Work out the finished part from the listing and answer in its coordinate system (mm). Face numbers are marked on the shaded views. Give positions to 0.01 mm unless a question says otherwise; leave off trailing zeros. Loops run counter-clockwise (first coordinate to the right, second up) from the corner with the lowest first, then second, coordinate; pieces in that order, holes last. Notation, with made-up numbers: (79, 27) - (108, 27) arc R11 ccw to (108, 35) - close; hole circle Ø7 at (-16, -10.5). An arc over 180 degrees is marked (long way). One line per item, written item: value.
from build123d import *

# Parameters (mm, degrees)
F0_W     = 40.64
F0_H     = 21.59
F1_DEPTH = 1.905
F2_R     = 5.08


with BuildPart() as f1:
    # F0 (on Front) → F1 (new body, symmetric)
    with BuildSketch(Plane.XZ):
        with Locations((-13.928885, -27.195361)):
            Rectangle(F0_W, F0_H)
    extrude(amount=F1_DEPTH, both=True)

    # F2
    f2_edges = [f1.edges().sort_by_distance(p)[0] for p in [
        (-34.248885, 0, -16.400361),
        (6.391115, 0, -16.400361),
        (-34.248885, 0, -37.990361),
        (6.391115, 0, -37.990361),
    ]]
    fillet(f2_edges, radius=F2_R)


solid = f1.part
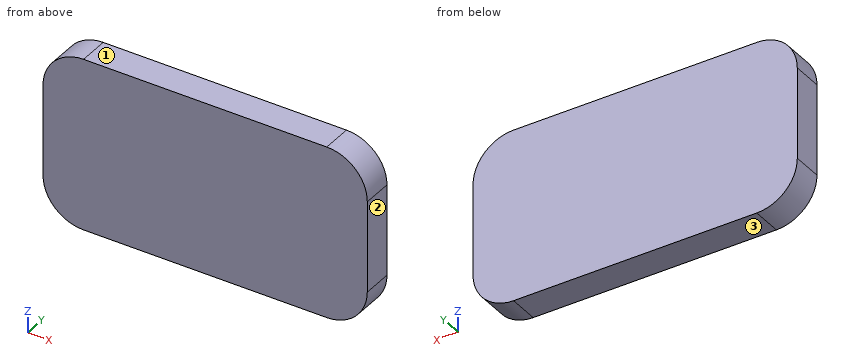
1. Section A-A (y = -0.5) is taken. Write down the section's boundary in (x, z).
Output:
outline: (-34.25, -32.91) arc R5.08 ccw to (-29.17, -37.99) - (1.31, -37.99) arc R5.08 ccw to (6.39, -32.91) - (6.39, -21.48) arc R5.08 ccw to (1.31, -16.4) - (-29.17, -16.4) arc R5.08 ccw to (-34.25, -21.48) - close
2. The mould has two halves that part along Z. Classify the marked faces 1, 2 and 3: released by +Z, released by -Z, zero draft, split by the parting line, or undercut.
Output:
face 1: released by +Z
face 2: zero draft
face 3: released by -Z
3. Find the intervals of material crossed by line 1 along Z through (x, y) = (1.5, -1.05); line 2 along X through (y, z) = (-0.35, -33); line 3 along X through (y, z) = (0.7, -34), in increasing order.
Output:
line 1: z = -37.99 to -16.4
line 2: x = -34.25 to 6.39
line 3: x = -34.13 to 6.27
4. Section B-B (z = -19.5) is taken. Write down the section's boundary in (x, y) (3 decimals), and give its area (3 significant figures).
Output:
outline: (-33.847, -1.905) - (5.989, -1.905) - (5.989, 1.905) - (-33.847, 1.905) - close
area: 152 mm²
